The model under review builds one solid part; all positions refer to its coordinate system, in mm. A direction names the side the tool comes from. Coordinates: 2 decimals unless noted, no trailing zeros. Order: outer loops, then holes, each group sorted by start corner. A loop starts at its lowest first (then second) coordinate and runs counter-clockwise, first axis right, second up. Notation, with made-up numbers: (67.5, 11) -> (87.5, 11) arc R28 ccw to (87.5, 32) -> close; hole circle Ø5 at (45.5, 17.25). An arc over 180 degrees is marked (long way). Put each result on its own line as item: value.
from build123d import *

# Parameters (mm, degrees)
SKETCH_1_R      = 1.5
EXTRUDE_1_DEPTH = 3
SKETCH_1_3_R    = 1.5
EXTRUDE_2_DEPTH = 3
EXTRUDE_3_DEPTH = 2


with BuildPart() as part:
    # Sketch 1 → Extrude 1 (new body)
    with BuildSketch(Plane.XY):
        with BuildLine():
            ThreePointArc((2.892953335, 0.590118878), (3.343078331, 0.126400512), (3.41560199, -0.515773572))
            ThreePointArc((3.41560199, -0.515773572), (2.785653548, -1.950535613), (1.652873302, -3.033211035))
            ThreePointArc((1.652873302, -3.033211035), (1.024622501, -3.18469756), (0.434917959, -2.920319445))
            Line((0.434917959, -2.920319445), (-1.978549256, -0.669724856))
            ThreePointArc((-1.978549256, -0.669724856), (-2.21171052, 1.548656378), (-0.047368195, 2.088287527))
            Line((-0.047368195, 2.088287527), (2.892953335, 0.590118878))
        make_face()
        Circle(SKETCH_1_R, mode=Mode.SUBTRACT)
        Circle(SKETCH_1_R)
    extrude(amount=EXTRUDE_1_DEPTH)

    # Sketch 1_3 → Extrude 2 (add)
    with BuildSketch(Plane.XY):
        Circle(SKETCH_1_3_R)
    extrude(amount=-EXTRUDE_2_DEPTH)

    # Sketch 2 → Extrude 3 (add)
    with BuildSketch(Plane(origin=(0, 0, -3), x_dir=(-1, 0, 0), z_dir=(0, 0, -1))):
        with BuildLine():
            Line((-2.439141124, 3.170266641), (-28.884678079, -17.176412053))
            ThreePointArc((-28.884678079, -17.176412053), (-29.408094987, -20.591769795), (-26.019689394, -21.268039933))
            Line((-26.019689394, -21.268039933), (2.144840772, -3.376337966))
            ThreePointArc((2.144840772, -3.376337966), (3.276608177, 2.294305745), (-2.439141124, 3.170266641))
        make_face()
    extrude(amount=EXTRUDE_3_DEPTH)


solid = part.part
Item 1: Consider section D-D on y = -5.75. Write out the cut boundary in (x, z).
Answers below:
outline: (1.59, -5) -> (14.03, -5) -> (14.03, -3) -> (1.59, -3) -> close
Item 2: For faces 5 (the cylindrical face through (2.8, -1.93, 1.48)), 6 (the flat face through (-0.755, -1.811, 1.479)), 7 (the flat face through (1.4, 1.35, 1.48)), 8 (the flat face through (12.135, -12.447, -3.986)), 9 (the cylindrical face through (1.034, -3.186, 1.479)), list the 3-axis set-ups (+Z, -Z, +X, -X, +Y, -Y) from which the entire face can be reached by the end or side of a thin tool; tool diameter is ignored.
Answers below:
face 5: +Z, +X, -Y
face 6: +Z, -X, -Y
face 7: +Z, +X, +Y
face 8: +Z, -Z, -X, -Y
face 9: +Z, -Y
Item 3: Consider section C-C on z = -1.75. Write out the cut boundary in (x, y), and give its area (3 significant figures).
Answers below:
outline: circle Ø3 at (0, 0)
area: 7.07 mm^2
Item 4: Mouldability with a two-part tool opening along Z and no side actions: class faces 1 (the cylindrical face through (29.438, -20.548, -3.986)), 2 (the cylindrical face through (-1.5, 0.07, -1.48)), 3 (the flat face through (1, -2, 0)), 4 (the flat face through (1, 0, 3)) as +Z half, -Z half, draft (parallel to the pull), parting line (faces both ways), or undercut.
Answers below:
face 1: draft
face 2: undercut
face 3: undercut
face 4: +Z half
Item 5: Consider section B-B on y = 1. Write out the cut boundary in (x, z).
Answers below:
outline: (-3.87, -5) -> (5.26, -5) -> (5.26, -3) -> (1.12, -3) -> (1.12, 0) -> (2.09, 0) -> (2.09, 3) -> (-2.46, 3) -> (-2.46, 0) -> (-1.12, 0) -> (-1.12, -3) -> (-3.87, -3) -> close
Item 6: For pin 1 Ø1 at (y, z) = (-5, -3) entering from +X; pin 2 Ø1 at (x, y) = (12.5, -6.5) entering from +Z, all flat-tipped, find the tip position at first contact; note any pin that passes through.
Answers below:
pin 1: x = 13.71
pin 2: z = -3
Item 7: For line 1 (Z direction, x = 13, y = -12.5); line 2 (Y direction, x = 1.5, z = 1); line 3 (X direction, y = -10, z = -3.25), list the stretches that pass through material, from the lowest coordinate up. Write a range as from..to.
Answers below:
line 1: -5..-3
line 2: -3.11..1.3
line 3: 8.28..19.56
Item 8: Consider section A-A on z = 2.25. Write out the cut boundary in (x, y).
Answers below:
outline: (-1.98, -0.67) -> (0.43, -2.92) arc R1 ccw to (1.65, -3.03) arc R4 ccw to (3.42, -0.52) arc R1 ccw to (2.89, 0.59) -> (-0.05, 2.09) arc R1.7 ccw to start
